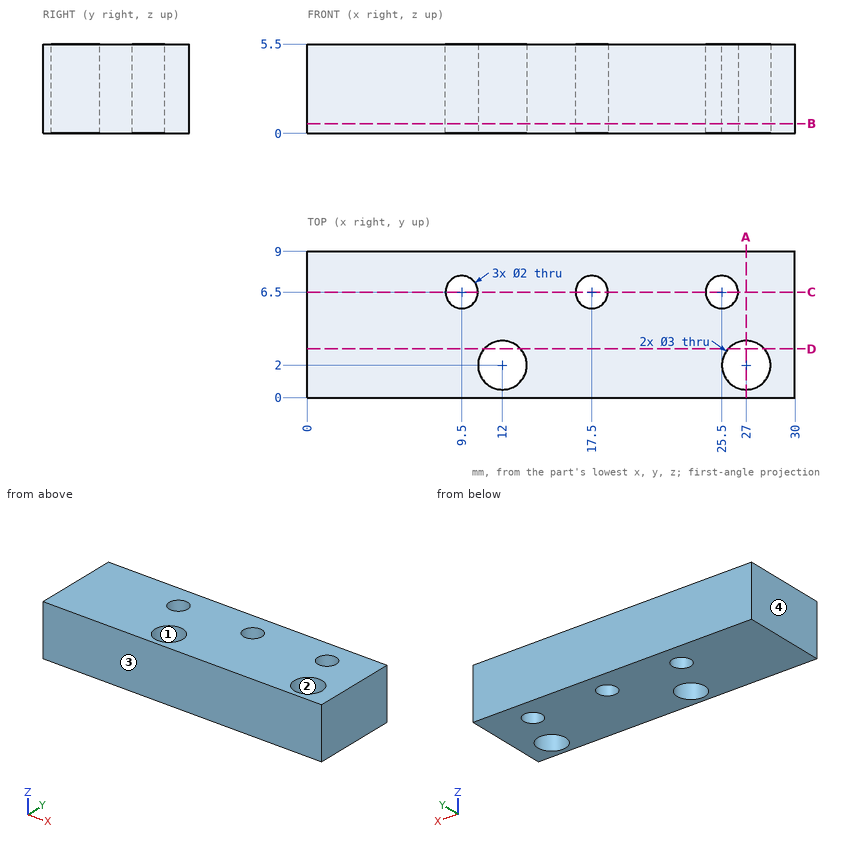
For this review, use the dimensioned drawing (mm, ordinates from the lowest corner) and the shaded views. Round coordinates to 2 decimals unless told otherwise and drop trailing zeros. Write each loop counter-clockwise with the first axis right and the second up, starting at its lowest first coordinate (ties: lowest second). Pieces come first, ordered by that corner, then holes. Notation, with made-up numbers: (62, 84.5) -> (97, 84.5) arc R22 ccw to (97, 123.5) -> close; hole circle Ø10 at (-36, -33.5). An arc over 180 degrees is marked (long way). Use one line per item in the form item = value.
Q1. Consider section B-B (z = 0.6). State the section outline as (x, y) points, then the cut area to 3 significant figures.
Resolved:
outline = (0, 0) -> (30, 0) -> (30, 9) -> (0, 9) -> close; hole circle Ø2 at (9.5, 6.5); hole circle Ø3 at (12, 2); hole circle Ø2 at (17.5, 6.5); hole circle Ø2 at (25.5, 6.5); hole circle Ø3 at (27, 2)
area = 246 mm²
Q2. Consider section C-C (y = 6.5). State the section outline as (x, z) points, then the cut area to 3 significant figures.
Resolved:
outline = (0, 0) -> (8.5, 0) -> (8.5, 5.5) -> (0, 5.5) -> close; (10.5, 0) -> (16.5, 0) -> (16.5, 5.5) -> (10.5, 5.5) -> close; (18.5, 0) -> (24.5, 0) -> (24.5, 5.5) -> (18.5, 5.5) -> close; (26.5, 0) -> (30, 0) -> (30, 5.5) -> (26.5, 5.5) -> close
area = 132 mm²
Q3. Consider section A-A (x = 27). State the section outline as (y, z) points, then the cut area to 3 significant figures.
Resolved:
outline = (0, 0) -> (0.5, 0) -> (0.5, 5.5) -> (0, 5.5) -> close; (3.5, 0) -> (9, 0) -> (9, 5.5) -> (3.5, 5.5) -> close
area = 33.0 mm²
Q4. The part is to be moulded in two halves that separate along Y. For the marked faces 1, 2, 3 and 4, say which applies: released by +Y, released by -Y, zero draft, split by the parting line, or undercut.
Resolved:
face_1 = undercut
face_2 = undercut
face_3 = released by -Y
face_4 = zero draft
Q5. Consider section D-D (y = 3). State the section outline as (x, z) points.
Resolved:
outline = (0, 0) -> (10.88, 0) -> (10.88, 5.5) -> (0, 5.5) -> close; (13.12, 0) -> (25.88, 0) -> (25.88, 5.5) -> (13.12, 5.5) -> close; (28.12, 0) -> (30, 0) -> (30, 5.5) -> (28.12, 5.5) -> close
Q6. To check wall thickness, follow probe 1 along Y at (x, z) = (17.5, 1.2); probe 2 along X at (y, z) = (7.25, 3.05); probe 3 along Y at (x, z) = (26.75, 2.9). State the ranges of each line that lie inside material, in increasing order. Write a range as from..to.
Resolved:
probe_1 = 0..5.5, 7.5..9
probe_2 = 0..8.84, 10.16..16.84, 18.16..24.84, 26.16..30
probe_3 = 0..0.52, 3.48..9
